Check sheet for the modelled part. Datum: model origin and axes. Units: mm. Round coordinates to 2 decimals unless told otherwise and drop trailing zeros. Loops run counter-clockwise (first coordinate to the right, second up) from the corner with the lowest first, then second, coordinate; pieces in that order, holes last. Notation, with made-up numbers: M -22.75,54.5 L 27.25,54.5 A22 ccw 27.25,88.5 Z; hole C 48.25,-11.5 d4. An arc over 180 degrees is marked long. Write item = value, one per line. Start each with the question number.
(1) Scan lines: L1, parallel to X at y = -23.5, z = 179; L2, parallel to X at y = -17, z = 138; L3, parallel to Z at x = -17, y = -1.25. Record each from-to range of solid material in increasing order. Write a range as from..to.
(2) Cross-section at B-B on y = -16. State how many separate pieces and enclosed holes the cut face has, plus the area to 3 significant figures.
(3) Mould release check, pull along Z, two halves, no side actions. Record for faces 1 (the face through (-101.5, -12.88, 79.24)), 2 (the face through (-80.11, -12.88, 21.2)), 3 (the face through (-71, 0, 135)), 4 (the face through (-58, -13, 0)): pulls with the +Z half, pulls with the -Z half, needs draft (parallel to the pull), parting line crosses it, or undercut.
(4) Cross-section at A-A on z = 91.5. Record the boundary of the cut face in (x, y), plus the area to 3 significant figures.
(5) Cross-section at C-C on z = 35.5. Record the boundary of the cut face in (x, y).
(6) Go/stop test with a flat-tipped pin: P1, Ø1.5, axis at x = -101.5, z = 215, coming from the +Y side. Record where the tip stops, or that it passes through.
from build123d import *

# Parameters (mm, degrees)
F0_W     = 114.3
F0_H     = 266.7
F1_DEPTH = 25.4
F2_R     = 3.175
F2_R_2   = 6.35
F2_R_3   = 9.525
F2_R_4   = 12.7
F2_R_5   = 15.875
F2_R_6   = 19.05
F3_DEPTH = 25.4
F5_DEPTH = 25.4


with BuildPart() as f1:
    # F0 (on Front) → F1 (new body)
    with BuildSketch(Plane.XZ):
        with Locations((-57.15, 133.35)):
            Rectangle(F0_W, F0_H)
    extrude(amount=F1_DEPTH)

    # F2 (on face) → F3 (cut)
    with BuildSketch(Plane.XZ.offset(25.4)):
        with BuildLine():
            ThreePointArc((-25.4, 57.15), (-44.45, 38.1), (-25.4, 19.05))
            Line((-25.4, 19.05), (-25.4, 38.1))
            Line((-25.4, 38.1), (-25.4, 57.15))
        make_face()
        with BuildLine():
            ThreePointArc((-25.4, 231.775), (-28.575, 228.6), (-25.4, 225.425))
            Line((-25.4, 225.425), (-25.4, 228.6))
            Line((-25.4, 228.6), (-25.4, 231.775))
        make_face()
        with BuildLine():
            Line((-25.4, 228.6), (-25.4, 225.425))
            ThreePointArc((-25.4, 225.425), (-23.154936, 226.354936), (-22.225, 228.6))
            ThreePointArc((-22.225, 228.6), (-23.154936, 230.845064), (-25.4, 231.775))
            Line((-25.4, 231.775), (-25.4, 228.6))
        make_face()
        with BuildLine():
            ThreePointArc((-25.4, 209.55), (-31.75, 203.2), (-25.4, 196.85))
            Line((-25.4, 196.85), (-25.4, 203.2))
            Line((-25.4, 203.2), (-25.4, 209.55))
        make_face()
        with BuildLine():
            Line((-25.4, 203.2), (-25.4, 196.85))
            ThreePointArc((-25.4, 196.85), (-20.909872, 198.709872), (-19.05, 203.2))
            ThreePointArc((-19.05, 203.2), (-20.909872, 207.690128), (-25.4, 209.55))
            Line((-25.4, 209.55), (-25.4, 203.2))
        make_face()
        with BuildLine():
            ThreePointArc((-25.4, 180.975), (-34.925, 171.45), (-25.4, 161.925))
            Line((-25.4, 161.925), (-25.4, 171.45))
            Line((-25.4, 171.45), (-25.4, 180.975))
        make_face()
        with BuildLine():
            Line((-25.4, 171.45), (-25.4, 161.925))
            ThreePointArc((-25.4, 161.925), (-18.664808, 164.714808), (-15.875, 171.45))
            ThreePointArc((-15.875, 171.45), (-18.664808, 178.185192), (-25.4, 180.975))
            Line((-25.4, 180.975), (-25.4, 171.45))
        make_face()
        with BuildLine():
            ThreePointArc((-25.4, 146.05), (-38.1, 133.35), (-25.4, 120.65))
            Line((-25.4, 120.65), (-25.4, 133.35))
            Line((-25.4, 133.35), (-25.4, 146.05))
        make_face()
        with BuildLine():
            Line((-25.4, 133.35), (-25.4, 120.65))
            ThreePointArc((-25.4, 120.65), (-16.419744, 124.369744), (-12.7, 133.35))
            ThreePointArc((-12.7, 133.35), (-16.419744, 142.330256), (-25.4, 146.05))
            Line((-25.4, 146.05), (-25.4, 133.35))
        make_face()
        with BuildLine():
            ThreePointArc((-25.4, 104.775), (-41.275, 88.9), (-25.4, 73.025))
            Line((-25.4, 73.025), (-25.4, 88.9))
            Line((-25.4, 88.9), (-25.4, 104.775))
        make_face()
        with BuildLine():
            Line((-25.4, 88.9), (-25.4, 73.025))
            ThreePointArc((-25.4, 73.025), (-14.17468, 77.67468), (-9.525, 88.9))
            ThreePointArc((-9.525, 88.9), (-14.17468, 100.12532), (-25.4, 104.775))
            Line((-25.4, 104.775), (-25.4, 88.9))
        make_face()
        with BuildLine():
            Line((-25.4, 38.1), (-25.4, 19.05))
            ThreePointArc((-25.4, 19.05), (-11.929616, 24.629616), (-6.35, 38.1))
            ThreePointArc((-6.35, 38.1), (-11.929616, 51.570384), (-25.4, 57.15))
            Line((-25.4, 57.15), (-25.4, 38.1))
        make_face()
        with Locations((-88.9, 228.6)):
            Circle(F2_R)
        with Locations((-88.9, 203.2)):
            Circle(F2_R_2)
        with Locations((-88.9, 171.45)):
            Circle(F2_R_3)
        with Locations((-88.9, 133.35)):
            Circle(F2_R_4)
        with Locations((-88.9, 88.9)):
            Circle(F2_R_5)
        with Locations((-88.9, 38.1)):
            Circle(F2_R_6)
    extrude(amount=-F3_DEPTH, mode=Mode.SUBTRACT)

    # F4 (on face) → F5 (cut)
    with BuildSketch(Plane.XZ.offset(25.4)):
        with BuildLine():
            ThreePointArc((-57.15, 260.35), (-76.2, 241.3), (-57.15, 222.25))
            Line((-57.15, 222.25), (-57.15, 241.3))
            Line((-57.15, 241.3), (-57.15, 260.35))
        make_face()
        with BuildLine():
            Line((-57.15, 241.3), (-57.15, 222.25))
            ThreePointArc((-57.15, 222.25), (-43.679616, 227.829616), (-38.1, 241.3))
            ThreePointArc((-38.1, 241.3), (-43.679616, 254.770384), (-57.15, 260.35))
            Line((-57.15, 260.35), (-57.15, 241.3))
        make_face()
        with BuildLine():
            ThreePointArc((-57.15, 217.4875), (-74.6125, 200.025), (-57.15, 182.5625))
            Line((-57.15, 182.5625), (-57.15, 200.025))
            Line((-57.15, 200.025), (-57.15, 217.4875))
        make_face()
        with BuildLine():
            Line((-57.15, 200.025), (-57.15, 182.5625))
            ThreePointArc((-57.15, 182.5625), (-44.802148, 187.677148), (-39.6875, 200.025))
            ThreePointArc((-39.6875, 200.025), (-44.802148, 212.372852), (-57.15, 217.4875))
            Line((-57.15, 217.4875), (-57.15, 200.025))
        make_face()
        with BuildLine():
            ThreePointArc((-57.15, 177.8), (-73.025, 161.925), (-57.15, 146.05))
            Line((-57.15, 146.05), (-57.15, 161.925))
            Line((-57.15, 161.925), (-57.15, 177.8))
        make_face()
        with BuildLine():
            Line((-57.15, 161.925), (-57.15, 146.05))
            ThreePointArc((-57.15, 146.05), (-45.92468, 150.69968), (-41.275, 161.925))
            ThreePointArc((-41.275, 161.925), (-45.92468, 173.15032), (-57.15, 177.8))
            Line((-57.15, 177.8), (-57.15, 161.925))
        make_face()
        with BuildLine():
            ThreePointArc((-57.15, 141.2875), (-71.4375, 127), (-57.15, 112.7125))
            Line((-57.15, 112.7125), (-57.15, 127))
            Line((-57.15, 127), (-57.15, 141.2875))
        make_face()
        with BuildLine():
            Line((-57.15, 127), (-57.15, 112.7125))
            ThreePointArc((-57.15, 112.7125), (-47.047212, 116.897212), (-42.8625, 127))
            ThreePointArc((-42.8625, 127), (-47.047212, 137.102788), (-57.15, 141.2875))
            Line((-57.15, 141.2875), (-57.15, 127))
        make_face()
        with BuildLine():
            ThreePointArc((-57.15, 107.95), (-69.85, 95.25), (-57.15, 82.55))
            Line((-57.15, 82.55), (-57.15, 95.25))
            Line((-57.15, 95.25), (-57.15, 107.95))
        make_face()
        with BuildLine():
            Line((-57.15, 95.25), (-57.15, 82.55))
            ThreePointArc((-57.15, 82.55), (-48.169744, 86.269744), (-44.45, 95.25))
            ThreePointArc((-44.45, 95.25), (-48.169744, 104.230256), (-57.15, 107.95))
            Line((-57.15, 107.95), (-57.15, 95.25))
        make_face()
        with BuildLine():
            ThreePointArc((-57.15, 77.7875), (-68.2625, 66.675), (-57.15, 55.5625))
            Line((-57.15, 55.5625), (-57.15, 66.675))
            Line((-57.15, 66.675), (-57.15, 77.7875))
        make_face()
        with BuildLine():
            Line((-57.15, 66.675), (-57.15, 55.5625))
            ThreePointArc((-57.15, 55.5625), (-49.292276, 58.817276), (-46.0375, 66.675))
            ThreePointArc((-46.0375, 66.675), (-49.292276, 74.532724), (-57.15, 77.7875))
            Line((-57.15, 77.7875), (-57.15, 66.675))
        make_face()
        with BuildLine():
            ThreePointArc((-57.15, 50.8), (-66.675, 41.275), (-57.15, 31.75))
            Line((-57.15, 31.75), (-57.15, 41.275))
            Line((-57.15, 41.275), (-57.15, 50.8))
        make_face()
        with BuildLine():
            Line((-57.15, 41.275), (-57.15, 31.75))
            ThreePointArc((-57.15, 31.75), (-50.414808, 34.539808), (-47.625, 41.275))
            ThreePointArc((-47.625, 41.275), (-50.414808, 48.010192), (-57.15, 50.8))
            Line((-57.15, 50.8), (-57.15, 41.275))
        make_face()
        with BuildLine():
            ThreePointArc((-49.2125, 19.05), (-51.53734, 24.66266), (-57.15, 26.9875))
            ThreePointArc((-57.15, 26.9875), (-62.76266, 13.43734), (-49.2125, 19.05))
        make_face()
    extrude(amount=-F5_DEPTH, mode=Mode.SUBTRACT)


solid = f1.part
Result:
q1.L1 = -114.3..-94.71, -83.09..-31.21, -19.59..0
q1.L2 = -114.3..-100.72, -77.08..-66.27, -48.03..-37.22, -13.58..0
q1.L3 = 0..21, 55.2..75.43, 102.37..123.82, 142.88..166.96, 175.94..266.7
q2.separate_pieces = 1
q2.enclosed_holes = 20
q2.area = 19,800 mm^2
q3.face_1 = undercut
q3.face_2 = undercut
q3.face_3 = needs draft
q3.face_4 = pulls with the -Z half
q4.outline = M -114.3,-25.4 L -104.56,-25.4 L -104.56,0 L -114.3,0 Z; M -73.24,-25.4 L -69.28,-25.4 L -69.28,0 L -73.24,0 Z; M -45.02,-25.4 L -41.06,-25.4 L -41.06,0 L -45.02,0 Z; M -9.74,-25.4 L 0,-25.4 L 0,0 L -9.74,0 Z
q4.area = 696 mm^2
q5.outline = M -114.3,-25.4 L -107.77,-25.4 L -107.77,0 L -114.3,0 Z; M -70.03,-25.4 L -64.72,-25.4 L -64.72,0 L -70.03,0 Z; M -49.58,-25.4 L -44.27,-25.4 L -44.27,0 L -49.58,0 Z; M -6.53,-25.4 L 0,-25.4 L 0,0 L -6.53,0 Z
q6.P1 = 0
